Model file for the job. Use its own axes, mm. Face numbers are marked on the shaded views. A direction names the side the tool comes from. Round coordinates to 2 decimals unless told otherwise and drop trailing zeros. Order: outer loops, then holes, each group sorted by start corner. A loop starts at its lowest first (then second) coordinate and runs counter-clockwise, first axis right, second up. Notation, with made-up numbers: (2.25, 12.25) - (48.25, 12.25) arc R30 ccw to (48.25, 36.25) - close; hole circle Ø11 at (88, 53.25). An arc over 180 degrees is marked (long way). Use one line per item in the form item = value.
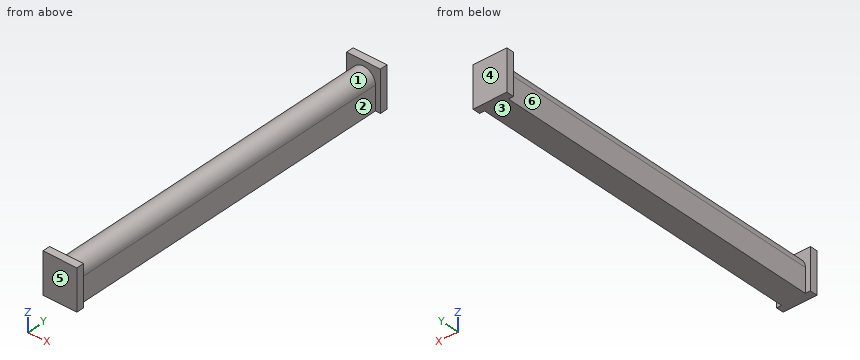
from build123d import *

# Parameters (mm, degrees)
BOSS_EXTRUDE1_DEPTH = 135
SKETCH8_W           = 13.5
SKETCH8_H           = 16.25
BOSS_EXTRUDE4_DEPTH = 3
SKETCH9_W           = 13.5
SKETCH9_H           = 16.25
BOSS_EXTRUDE5_DEPTH = 3


with BuildPart() as part:
    # Sketch5 → Boss-Extrude1 (new body)
    with BuildSketch(Plane(origin=(0, 0, 0), x_dir=(1, 0, 0), z_dir=(0, 1, 0))):
        with BuildLine():
            Line((0, 0), (9.5, 0))
            Line((9.5, 0), (9.5, -9.5))
            ThreePointArc((9.5, -9.5), (4.75, -14.25), (0, -9.5))
            Line((0, -9.5), (0, 0))
        make_face()
    extrude(amount=-BOSS_EXTRUDE1_DEPTH)

    # Sketch8 → Boss-Extrude4 (add)
    with BuildSketch(Plane.XZ.offset(135)):
        with Locations((4.75, 8.125)):
            Rectangle(SKETCH8_W, SKETCH8_H)
    extrude(amount=BOSS_EXTRUDE4_DEPTH)

    # Sketch9 → Boss-Extrude5 (add)
    with BuildSketch(Plane(origin=(0, 0, 0), x_dir=(1, 0, 0), z_dir=(0, 1, 0))):
        with Locations((4.75, -8.125)):
            Rectangle(SKETCH9_W, SKETCH9_H)
    extrude(amount=BOSS_EXTRUDE5_DEPTH)


solid = part.part
(1) Pin check, flat tips, straight feed: pin 1 (1.5 mm diameter, centred on x = 5.5, y = -18, fed in from -Z); pin 2 (3 mm diameter, centred on y = -57.5, z = 8.5, fed in from -X); pin 3 (1.5 mm diameter, centred on y = -117, z = 5, fed in from +X). Stop position of each tip, or through.
Report:
pin_1 = 0
pin_2 = 0
pin_3 = 9.5
(2) Pull direction Y, two halves, no side cores. Call the marked faces 3, 4, 5 and 6: released by +Y, released by -Y, zero draft, split by the parting line, or undercut.
Report:
face_3 = zero draft
face_4 = released by +Y
face_5 = released by -Y
face_6 = undercut
(3) Probe probe 1 along Y at (x, z) = (-0.25, 11.25); probe 2 along X at (y, z) = (-46, 5.25); probe 3 along Z at (x, y) = (4.5, -95.5). List the from-to ranges inside material, lowest first. Write a range as [from, to].
Report:
probe_1 = [-138, -135], [0, 3]
probe_2 = [0, 9.5]
probe_3 = [0, 14.24]
(4) Slice it at A-A on z = 4. Give the cut face in (x, y), then the cut area to 3 significant figures.
Report:
outline = (-2, -138) - (11.5, -138) - (11.5, -135) - (9.5, -135) - (9.5, 0) - (11.5, 0) - (11.5, 3) - (-2, 3) - (-2, 0) - (0, 0) - (0, -135) - (-2, -135) - close
area = 1,360 mm2
(5) Slice it at B-B on x = 4.75. Give the cut face in (y, z), then the cut area to 3 significant figures.
Report:
outline = (-138, 0) - (3, 0) - (3, 16.25) - (0, 16.25) - (0, 14.25) - (-135, 14.25) - (-135, 16.25) - (-138, 16.25) - close
area = 2,020 mm2
(6) Tool access for the marked faces 1 and 2: list every direction of +Z, -Z, +X, -X, +Y, -Y with a clear straight run to the whole face (end or side of a thin tool).
Report:
face_1 = +Z
face_2 = +Z, -Z, +X
(7) Slice it at C-C on y = -84. Give the cut face in (x, z), then the cut area to 3 significant figures.
Report:
outline = (0, 0) - (9.5, 0) - (9.5, 9.5) arc R4.75 ccw to (0, 9.5) - close
area = 126 mm2
